from build123d import *

# Parameters (mm, degrees)
EXTRUDE_1_DEPTH              = 32
EXTRUDE_1_DEPTH_BACK         = 32
SKETCH_1_R                   = 4
HOLE_WIZARD_M3_2_D           = 2.5
HOLE_WIZARD_M3_2_CSINK_D     = 3.05
HOLE_WIZARD_M3_2_CSINK_ANGLE = 90
SKETCH_18_W                  = 33.250745193
SKETCH_18_H                  = 19.055234746
SKETCH_18_W_2                = 46.103437085
SKETCH_18_H_2                = 35.552719861
CUT_EXTRUDE_1_DEPTH          = 7
CUT_EXTRUDE_2_DEPTH          = 12
CUT_EXTRUDE_START            = -12
CUT_EXTRUDE_3_DEPTH          = 12


with BuildPart() as part:
    # Sketch 1 → Extrude 1 (new, two sides: drawn at the far end of the back side and taken through both)
    with BuildSketch(Plane(origin=(0, 0, 0), x_dir=(1, 0, 0), z_dir=(0, 1, 0)).offset(-EXTRUDE_1_DEPTH_BACK)):
        with Locations(Location((0, 0, 0), (0, 0, 270))):
            Circle(SKETCH_1_R)
    extrude(amount=EXTRUDE_1_DEPTH + EXTRUDE_1_DEPTH_BACK)

    # Hole Wizard M3 _2 (through all)
    with Locations(Plane(origin=(10, 0, 0), x_dir=(0, 0, -1), z_dir=(1, 0, 0))):
        with Locations((0, 28), (0, -28)):
            CounterSinkHole(HOLE_WIZARD_M3_2_D / 2, HOLE_WIZARD_M3_2_CSINK_D / 2, counter_sink_angle=HOLE_WIZARD_M3_2_CSINK_ANGLE)

    # Sketch 18 → Cut-Extrude 1 (cut)
    with BuildSketch(Plane(origin=(10, 0, 0), x_dir=(0, 0, -1), z_dir=(1, 0, 0))):
        with Locations((-0.619455311, 29.527617373)):
            Rectangle(SKETCH_18_W, SKETCH_18_H)
        with Locations((-0.267764737, -37.77635993)):
            Rectangle(SKETCH_18_W_2, SKETCH_18_H_2)
    extrude(amount=-CUT_EXTRUDE_1_DEPTH, mode=Mode.SUBTRACT)

    # Sketch 19 → Cut-Extrude 2 (cut)
    with BuildSketch(Plane.XZ.offset(32)):
        with BuildLine():
            Line((3, -2.645751311), (3, 2.645751311))
            ThreePointArc((3, 2.645751311), (4, 0), (3, -2.645751311))
        make_face()
        with BuildLine():
            Line((-3, -2.645751311), (-3, 2.645751311))
            ThreePointArc((-3, 2.645751311), (-4, 0), (-3, -2.645751311))
        make_face()
    extrude(amount=-CUT_EXTRUDE_2_DEPTH, mode=Mode.SUBTRACT)

    # Sketch 20 → Cut-Extrude 3 (cut)
    with BuildSketch(Plane(origin=(0, 32, 0), x_dir=(1, 0, 0), z_dir=(0, 1, 0)).offset(CUT_EXTRUDE_START)):
        with BuildLine():
            Line((3, -2.645751311), (3, 2.645751311))
            ThreePointArc((3, 2.645751311), (4, 0), (3, -2.645751311))
        make_face()
        with BuildLine():
            Line((-3, -2.645751311), (-3, 2.645751311))
            ThreePointArc((-3, 2.645751311), (-4, 0), (-3, -2.645751311))
        make_face()
    extrude(amount=CUT_EXTRUDE_3_DEPTH, mode=Mode.SUBTRACT)


solid = part.part
Can you work these out from the model? Positions are in its coordinate system, mm. A direction names the side the tool comes from. Coordinates: 2 decimals unless noted, no trailing zeros. Loops run counter-clockwise (first coordinate to the right, second up) from the corner with the lowest first, then second, coordinate; pieces in that order, holes last. Notation, with made-up numbers: (-6.5, 30.25) - (51.5, 30.25) arc R23 ccw to (51.5, 63.25) - close; hole circle Ø5 at (-26.75, 32.25). An arc over 180 degrees is marked (long way). Put each result on its own line as item: value. Start each with the question number.
Item 1: Suppose I cut it at A-A (z = 0). Please give me the cut outline in (x, y).
Item 2: If I drill on line 1 along Y through (x, z) = (0.1, 0); line 2 along Y through (x, z) = (-3.25, -2); line 3 along X through (y, z) = (10, 3), over which ranges is the centre line in solid material (lowest first)?
Item 3: Suppose I cut it at B-B (x = 0). Please give me the cut outline in (y, z), and give its area (3 significant figures).
Item 4: For pin 1 (0.8 mm diameter, centred on x = 3.5, z = 0.5, fed in from +Y); pin 2 (1 mm diameter, centred on x = 2.5, y = -18.5, fed in from +Z); pin 3 (1.6 mm diameter, centred on y = 23.5, z = 0, fed in from -X), each with a flat end and sliding along its axis, tell me the tip position at first contact or that it passes through.
Item 5: Suppose I cut it at D-D (y = 2.5). Please give me the cut outline in (x, z).
Item 6: If we mould it in two halves opening along Y, with no side actions, what happens to faces 5 (the face through (-3, 26, 0)), 6 (the face through (0, -32, 0)), 7 (the face through (-0.04, 26.78, -0.27))? For each: +Y half, -Y half, draft (parallel to the pull), parting line (faces both ways), or undercut.
Item 7: Suppose I cut it at C-C (y = 28). Please give me the cut outline in (x, z).
Item 8: Which directions (+Z, -Z, +X, -X, +Y, -Y) give clear straight access to the entire face, cutting with the end or side of a thin tool? Please do faces 1 (the face through (-3.4, 20, 0)), 2 (the face through (-3.4, -20, 0)), 3 (the face through (3.4, 20, 0)), 4 (the face through (3.4, -20, 0)).
Here are the results:
1. outline: (-4, -20) - (-3, -20) - (-3, -26.75) - (3, -26.75) - (3, -20) - (4, -20) - (4, 20) - (3, 20) - (3, 26.75) - (-3, 26.75) - (-3, 20) - (-4, 20) - close; (-3, -32) - (3, -32) - (3, -29.25) - (-3, -29.25) - close; (-3, 29.25) - (3, 29.25) - (3, 32) - (-3, 32) - close
2. line 1: -32 to -29.25, -26.75 to 26.75, 29.25 to 32
2. line 2: -20 to 20
2. line 3: -2.65 to 2.65
3. outline: (-32, -4) - (32, -4) - (32, 4) - (-32, 4) - close; hole circle Ø2.5 at (-28, 0); hole circle Ø2.5 at (28, 0)
3. area: 502 mm²
4. pin 1: y = 20
4. pin 2: z = 3.46
4. pin 3: x = -3
5. outline: circle Ø8 at (0, 0)
6. face 5: draft
6. face 6: -Y half
6. face 7: undercut
7. outline: (-3, -2.65) arc R4 ccw to (3, -2.65) - (3, -1.25) - (-3, -1.25) - close; (-3, 1.25) - (3, 1.25) - (3, 2.65) arc R4 ccw to (-3, 2.65) - close
8. face 1: +Z, -Z, -X, +Y
8. face 2: +Z, -Z, -X, -Y
8. face 3: +Z, -Z, +X, +Y
8. face 4: +Z, -Z, +X, -Y
